from build123d import *

# Parameters (mm, degrees)
BOSS_EXTRUDE1_DEPTH = 20
FILLET1_R           = 50
FILLET2_R           = 50
FILLET3_R           = 5
FILLET4_R           = 10
FILLET5_R           = 1
FILLET6_R           = 1


with BuildPart() as part:
    # Sketch1 → Boss-Extrude1 (new body)
    with BuildSketch(Plane.XY):
        with BuildLine():
            Line((1.53e-15, -7.5), (81.46535975563725, -15))
            ThreePointArc((81.46535975563725, -15), (95.96612319887386, -3.8376893521092743), (88.88528315077919, 13.036285391560943))
            Line((88.88528315077919, 13.036285391560943), (73.17379777974874, 12.49999999999999))
            Line((73.17379777974874, 12.49999999999999), (58.74284079566012, 9.013925925539251))
            Line((58.74284079566012, 9.013925925539251), (43.44024523082493, 10.4682923771142))
            Line((43.44024523082493, 10.4682923771142), (43.44024523082493, 7.968292377114199))
            Line((43.44024523082493, 7.968292377114199), (58.74284079566012, 6.51392592553925))
            Line((58.74284079566012, 6.51392592553925), (74.04543636049529, 10.059559473964299))
            Line((74.04543636049529, 10.059559473964299), (88.88528315077919, 10.059559473964299))
            ThreePointArc((88.88528315077919, 10.059559473964299), (93.33958590778194, -3.9054773444129744), (81.46535975563725, -12.49999999999999))
            Line((81.46535975563725, -12.49999999999999), (-7.7e-16, -5))
            Line((-7.7e-16, -5), (1.53e-15, -7.5))
        make_face()
    extrude(amount=BOSS_EXTRUDE1_DEPTH)

    # Fillet1
    fillet1_edges = [part.edges().sort_by_distance(p)[0] for p in [
        (58.74284079566012, 9.013925925539251, 10),
        (73.17379777974874, 12.49999999999999, 10),
    ]]
    fillet(fillet1_edges, radius=FILLET1_R)

    # Fillet2
    fillet2_edges = [part.edges().sort_by_distance(p)[0] for p in [
        (74.04543636049529, 10.059559473964299, 10),
        (58.74284079566012, 6.51392592553925, 10),
    ]]
    fillet(fillet2_edges, radius=FILLET2_R)

    # Fillet3
    fillet3_edges = [part.edges().sort_by_distance(p)[0] for p in [
        (88.88528315077919, 10.059559473964299, 10),
        (88.88528315077919, 13.036285391560945, 10),
    ]]
    fillet(fillet3_edges, radius=FILLET3_R)

    # Fillet4
    # the kernel refuses this fillet: 10 mm, written as the material it adds along each edge
    with BuildSketch(Plane(origin=(81.46535975563725, -12.499999999999993, 0), x_dir=(0.9983825762287738, 0.05685271746184882, 0), z_dir=(0, 0, 1))) as fillet4_piece_1:
        with BuildLine():
            CenterArc((0.8527907619277444, 9.983825762287736), FILLET4_R, 261.4807895615496, 11.77838854979251)
            Line((-0.6286192920357523, 0.09416326794467102), (0, 0))
            ThreePointArc((0, 0), (0.7106589682731511, -0.02021779714032781), (1.4213179365462814, 1e-17))
        make_face()
    extrude(amount=20)
    # the kernel refuses this fillet: 10 mm, written as the material it takes off along each edge
    with BuildSketch(Plane(origin=(81.46535975563715, -14.999999999999993, -2.523941837712784), x_dir=(-0.9957888906378437, 0.09167597985433422, 0), z_dir=(0, 0, 1))) as fillet4_2_piece_1:
        with BuildLine():
            CenterArc((0.5828793997689569, -10), FILLET4_R, 90.00000000000003, 9.11705963897387)
            ThreePointArc((-1.0016411963229432, -0.12633328086467327), (-0.5018837587629004, -0.05473730613968529), (0, 0))
            Line((0, 0), (0.5828793997689534, 0))
        make_face()
    extrude(amount=25.047883675425567, mode=Mode.SUBTRACT)

    # Fillet5
    fillet5_edges = [part.edges().sort_by_distance(p)[0] for p in [
        (1.53e-15, -7.5, 10),
        (-7.7e-16, -5, 10),
        (43.44024523082493, 7.968292377114199, 10),
        (43.44024523082493, 10.4682923771142, 10),
    ]]
    fillet(fillet5_edges, radius=FILLET5_R)

    # Fillet6
    fillet6_edges = [part.edges().sort_by_distance(p)[0] for p in [
        (67.55312596624809, 11.142219063385667, 0),
        (67.55312596624809, 11.142219063385667, 20),
        (82.78750373367262, 12.828147844719894, 0),
        (73.2087271321753, 12.243940169804823, 0),
        (82.78750373367262, 12.828147844719894, 20),
        (73.2087271321753, 12.243940169804823, 20),
        (58.69337304228126, 9.708148200467306, 0),
        (58.69337304228126, 9.708148200467306, 20),
        (83.38196474552188, 10.059559473964299, 0),
        (83.38196474552188, 10.059559473964299, 20),
        (67.57035497563798, 8.559273742065987, 0),
        (67.57035497563798, 8.559273742065987, 20),
        (58.69921223462093, 7.16938370928515, 0),
        (58.69921223462093, 7.16938370928515, 20),
        (74.08244123035955, 9.73590992988975, 0),
        (74.08244123035955, 9.73590992988975, 20),
        (88.99028016615965, 12.753456202652604, 0),
        (88.99028016615965, 12.753456202652604, 20),
        (89.0184612808635, 9.634775220054735, 0),
        (89.0184612808635, 9.634775220054735, 20),
        (95.84204739674057, -4.27911818838268, 0),
        (95.84204739674057, -4.27911818838268, 20),
        (93.17154749853181, -4.383510981862012, 0),
        (81.6792624975188, -14.987925542926858, 0),
        (93.17154749853181, -4.383510981862012, 20),
        (81.6792624975188, -14.987925542926858, 20),
        (81.85897083662152, -12.483235942602048, 0),
        (81.85897083662152, -12.483235942602048, 20),
        (47.4966925492185, 7.582765564524983, 0),
        (47.4966925492185, 7.582765564524983, 20),
        (40.89662947245553, -11.265093801383376, 0),
        (4.7e-16, -6.342063670037142, 0),
        (40.96203987478691, -8.771115723080602, 0),
        (43.44024523082493, 9.123251869416467, 0),
        (47.471858609430626, 10.085125794770558, 0),
        (0.326084567565907, -5.3574840944297595, 0),
        (0.261191506595139, -7.2617501846737555, 0),
        (43.767420646607164, 10.108547727110885, 0),
        (43.70044317698066, 8.204933481348554, 0),
        (43.44024523082493, 9.123251869416467, 20),
        (40.89662947245553, -11.265093801383376, 20),
        (47.471858609430626, 10.085125794770558, 20),
        (40.96203987478691, -8.771115723080602, 20),
        (4.7e-16, -6.342063670037142, 20),
        (0.326084567565907, -5.3574840944297595, 20),
        (0.261191506595139, -7.2617501846737555, 20),
        (43.767420646607164, 10.108547727110885, 20),
        (43.70044317698066, 8.204933481348554, 20),
    ]]
    fillet(fillet6_edges, radius=FILLET6_R)


solid = part.part
Can you work these out from the model? Positions are in its coordinate system, mm. A direction names the side the tool comes from. Coordinates: 2 decimals unless noted, no trailing zeros. Write each loop counter-clockwise with the first axis right and the second up, starting at its lowest first coordinate (ties: lowest second). Pieces come first, ordered by that corner, then holes.
Q1. If we mould it in two halves opening along X, with no side actions, what happens to faces 6 (the face through (66.6, -12.4, 0)), 7 (the face through (47.569, 7.878, 19.715)), 8 (the face through (41.52, -8.823, 9.874))? For each: +X half, -X half, draft (parallel to the pull), parting line (faces both ways), or undercut.
Results found:
face 6: draft
face 7: -X half
face 8: undercut
Q2. Imagine slicing it at B-B, the plane y = 0. List the corners of the cut face in (x, z) for me.
Results found:
outline: (93.97, 1) arc R1 ccw to (94.97, 0) - (95.47, 0) arc R1 ccw to (96.47, 1) - (96.47, 19) arc R1 ccw to (95.47, 20) - (94.97, 20) arc R1 ccw to (93.97, 19) - close
Q3. Which directions (+Z, -Z, +X, -X, +Y, -Y) give clear straight access to the entire face, cutting with the end or side of a thin tool? Please do faces 1 (the face through (40.376, -9.019, 19.715)), 2 (the face through (47.402, 9.79, 19.715)), 3 (the face through (40.376, -9.019, 0.285)), 4 (the face through (47.402, 9.79, 0.285)), 5 (the face through (83, 10.06, 10)).
Results found:
face 1: +Z
face 2: +Z, +Y
face 3: -Z
face 4: -Z, +Y
face 5: +Z, -Z
Q4. Imagine slicing it at A-A, the plane z = 6. List the corners of the cut face in (x, y) for me, plus the area to 3 significant figures.
Results found:
outline: (0, -6.59) arc R1 ccw to (0.91, -7.58) - (80.88, -14.95) arc R10 ccw to (82.47, -14.97) arc R15 ccw to (90.49, 11.98) arc R5 ccw to (87.31, 12.98) - (78.26, 12.67) arc R50 ccw to (68.23, 11.3) - (66.88, 10.98) arc R50 cw to (50.41, 9.81) - (44.53, 10.36) arc R1 ccw to (43.44, 9.37) - (43.44, 8.88) arc R1 ccw to (44.35, 7.88) - (50.65, 7.28) arc R50 ccw to (66.66, 8.35) - (68.48, 8.77) arc R50 cw to (79.76, 10.06) - (87, 10.06) arc R5 cw to (90.69, 8.43) arc R12.5 cw to (82.88, -12.42) arc R10 cw to (80.83, -12.44) - (1.09, -5.1) arc R1 ccw to (0, -6.1) - close
area: 410 mm2
Q5. For P1, Ø6, axis at x = 86, y = -7.5, coming from the +Z side; P2, Ø4, axis at x = 25, z = 9, coming from the -Y side; P3, Ø1.5, axis at x = 72, z = 13, coming from the +Y side; P4, Ø2, axis at y = 8.5, z = 2, coming from the -X side, each with a flat end and sliding along its axis, tell me the tip position at first contact or that it passes through.
Results found:
P1: passes through
P2: stops at y = -9.99
P3: stops at y = 12.18
P4: stops at x = 43.44
Q6. Please list where these lines run through material, in increasing order: L1, parallel to Y at x = 69, z = 15.75; L2, parallel to Y at x = 62.5, z = 15; L3, parallel to Y at x = 16, z = 10.75.
Results found:
L1: y = -13.85 to -11.35, 8.89 to 11.49
L2: y = -13.25 to -10.75, 7.57 to 10.13
L3: y = -8.97 to -6.47
